```python
from build123d import *

# Parameters (mm, degrees)
SKETCH2_R           = 45.212
SKETCH2_R_2         = 32.258
BOSS_EXTRUDE3_DEPTH = 40.64
SKETCH4_R           = 32.258
BOSS_EXTRUDE4_DEPTH = 7.62
BOSS_EXTRUDE4_TAPER = 25
CUT_EXTRUDE1_DEPTH  = 81.10791158
SKETCH7_R           = 2.286
CUT_EXTRUDE2_DEPTH  = 81.107911519
BOSS_EXTRUDE8_START = -7.62
BOSS_EXTRUDE8_DEPTH = 11.684
SKETCH18_R          = 8.567257543
CUT_EXTRUDE3_DEPTH  = 5.08
SKETCH19_R          = 2.286
CUT_EXTRUDE4_DEPTH  = 85.454467418
BOSS_EXTRUDE9_START = -15.24
BOSS_EXTRUDE9_DEPTH = 15.24
CUT_EXTRUDE5_START  = -28.956
SKETCH21_R          = 2.286
CUT_EXTRUDE5_DEPTH  = 28.956
CIRPATTERN1_COUNT   = 2
CUT_EXTRUDE6_DEPTH  = 91.648631066


with BuildPart() as part:
    # Sketch2 → Boss-Extrude3 (new body)
    # profile 1 of 2: a face of its own
    with BuildSketch(Plane(origin=(0, 0, 0), x_dir=(1, 0, 0), z_dir=(0, 1, 0))):
        with Locations(Location((0, 0, 0), (0, 0, 270))):
            Circle(SKETCH2_R)
        Circle(SKETCH2_R_2, mode=Mode.SUBTRACT)
    # profile 2 of 2: a face of its own
    with BuildSketch(Plane(origin=(0, 0, 0), x_dir=(1, 0, 0), z_dir=(0, 1, 0))):
        Circle(SKETCH2_R_2)
        Polygon((0, 6.35), (-6.35, 3.483506942), (-6.35, -3.483506942), (0, -6.35), (6.35, -3.483506942), (6.35, 3.483506942), align=None, mode=Mode.SUBTRACT)
    extrude(amount=-BOSS_EXTRUDE3_DEPTH)

    # Sketch4 → Boss-Extrude4 (add)
    with BuildSketch(Plane(origin=(0, 0, 0), x_dir=(1, 0, 0), z_dir=(0, 1, 0))):
        Circle(SKETCH4_R)
    extrude(amount=BOSS_EXTRUDE4_DEPTH, taper=BOSS_EXTRUDE4_TAPER)

    # Sketch6 → Cut-Extrude1 (cut, through all)
    with BuildSketch(Plane(origin=(0, -40.64, 0), x_dir=(-1, 0, 0), z_dir=(0, -1, 0))):
        Polygon((6.35, -3.483506942), (0, -6.35), (-6.35, -3.483506942), (-6.35, 3.483506942), (0, 6.35), (6.35, 3.483506942), align=None)
    extrude(amount=-CUT_EXTRUDE1_DEPTH, mode=Mode.SUBTRACT)

    # Sketch7 → Cut-Extrude2 (cut, through all)
    with BuildSketch(Plane(origin=(0, 7.62, 0), x_dir=(1, 0, 0), z_dir=(0, 1, 0))):
        with Locations(Location((-16.495222192, 16.6624, 0), (0, 0, 270))):
            Circle(SKETCH7_R)
        with Locations(Location((16.6624, 16.6624, 0), (0, 0, 270))):
            Circle(SKETCH7_R)
        with Locations(Location((16.6624, -16.6624, 0), (0, 0, 270))):
            Circle(SKETCH7_R)
        with Locations(Location((-16.495222192, -16.6624, 0), (0, 0, 270))):
            Circle(SKETCH7_R)
    extrude(amount=-CUT_EXTRUDE2_DEPTH, mode=Mode.SUBTRACT)

    # Sketch12 → Boss-Extrude8 (add)
    with BuildSketch(Plane(origin=(0, 7.62, 0), x_dir=(1, 0, 0), z_dir=(0, 1, 0)).offset(BOSS_EXTRUDE8_START)):
        with BuildLine():
            ThreePointArc((-45.091998917, -3.291895759), (-45.888251869, -5.330050438), (-47.973633707, -5.992829324))
            ThreePointArc((-47.973633707, -5.992829324), (-61.102572974, -22.2395178), (-40.602051954, -26.246083736))
            ThreePointArc((-40.602051954, -26.246083736), (-38.578530729, -25.413344212), (-36.658465006, -26.462839746))
            ThreePointArc((-36.658465006, -26.462839746), (-42.485382771, -15.46341472), (-45.091998917, -3.291895759))
        make_face()
    extrude(amount=-BOSS_EXTRUDE8_DEPTH)

    # Sketch18 → Cut-Extrude3 (cut)
    with BuildSketch(Plane(origin=(0, 0, 0), x_dir=(1, 0, 0), z_dir=(0, 1, 0))):
        with Locations(Location((-49.645840541, -18.069608212, 0), (0, 0, 270))):
            Circle(SKETCH18_R)
    extrude(amount=-CUT_EXTRUDE3_DEPTH, mode=Mode.SUBTRACT)

    # Sketch19 → Cut-Extrude4 (cut, through all)
    with BuildSketch(Plane(origin=(0, -5.08, 0), x_dir=(1, 0, 0), z_dir=(0, 1, 0))):
        with Locations(Location((-49.645840541, -18.069608212, 0), (0, 0, 270))):
            Circle(SKETCH19_R)
    extrude(amount=-CUT_EXTRUDE4_DEPTH, mode=Mode.SUBTRACT)

    # Sketch20 → Boss-Extrude9 (add)
    with BuildSketch(Plane.XZ.offset(40.64).offset(BOSS_EXTRUDE9_START)):
        with BuildLine():
            ThreePointArc((42.485382852, -15.463414497), (44.831385262, -12.89196184), (48.307822394, -12.717373918))
            Line((48.307822394, -12.717373918), (61.237093085, -17.295868799))
            Line((61.237093085, -17.295868799), (62.000175566, -15.140990351))
            Line((62.000175566, -15.140990351), (60.601893265, -12.209430544))
            Line((60.601893265, -12.209430544), (44.72934622, -6.588666841))
            ThreePointArc((44.72934622, -6.588666841), (43.832551012, -11.082978649), (42.485382852, -15.463414497))
        make_face()
        with BuildLine():
            ThreePointArc((45.180509286, -21.309596065), (42.629626793, -18.941243028), (42.485382852, -15.463414497))
            ThreePointArc((42.485382852, -15.463414497), (40.701683588, -19.684966271), (38.499780526, -23.704257918))
            Line((38.499780526, -23.704257918), (54.271814253, -29.601179693))
            Line((54.271814253, -29.601179693), (57.22733096, -28.254273131))
            Line((57.22733096, -28.254273131), (58.027905034, -26.113040506))
            Line((58.027905034, -26.113040506), (45.180509286, -21.309596065))
        make_face()
    extrude(amount=BOSS_EXTRUDE9_DEPTH)

    # Sketch21 → Cut-Extrude5 (cut)
    # profile 1 of 2: a face of its own
    with BuildSketch(Plane.XZ.offset(40.64).offset(CUT_EXTRUDE5_START)):
        with BuildLine():
            Line((-20.08732464, 27.438707345), (-28.082012675, 35.43339538))
            ThreePointArc((-28.082012675, 35.43339538), (-31.885487137, 32.053715136), (-35.285134805, 28.268077504))
            Line((-35.285134805, 28.268077504), (-27.271504992, 20.254502449))
            Line((-27.271504992, 20.254502449), (-30.86360744, 16.662375455))
            Line((-30.86360744, 16.662375455), (-23.679427089, 9.478195103))
            ThreePointArc((-23.679427089, 9.478195103), (-9.311017295, 9.478195103), (-9.311017295, 23.846604897))
            Line((-9.311017295, 23.846604897), (-16.495222192, 31.030809794))
            Line((-16.495222192, 31.030809794), (-20.08732464, 27.438707345))
        make_face()
        with Locations(Location((-16.495222192, 16.6624, 0), (0, 0, 90))):
            Circle(SKETCH21_R, mode=Mode.SUBTRACT)
    # profile 2 of 2: a face of its own
    with BuildSketch(Plane.XZ.offset(40.64).offset(CUT_EXTRUDE5_START)):
        with BuildLine():
            ThreePointArc((16.6624, 26.8224), (6.5024, 16.6624), (16.6624, 6.5024))
            Line((16.6624, 6.5024), (26.8224, 6.5024))
            Line((26.8224, 6.5024), (26.8224, 11.844066963))
            Line((26.8224, 11.844066963), (43.63304965, 11.844066963))
            ThreePointArc((43.63304965, 11.844066963), (41.873887087, 17.050000709), (39.496151472, 22.004066963))
            Line((39.496151472, 22.004066963), (25.304864582, 22.004066963))
            Line((25.304864582, 22.004066963), (25.304864582, 26.8224))
            Line((25.304864582, 26.8224), (16.6624, 26.8224))
        make_face()
        with Locations(Location((16.6624, 16.6624, 0), (0, 0, 90))):
            Circle(SKETCH21_R, mode=Mode.SUBTRACT)
    cut_extrude5 = extrude(amount=CUT_EXTRUDE5_DEPTH, mode=Mode.SUBTRACT)

    # CirPattern1: Cut-Extrude5 ×2 about axis
    cirpattern1_axis = Axis((0, 0, 0), (0, 1, 0))
    for i in range(1, CIRPATTERN1_COUNT):
        add(cut_extrude5.rotate(cirpattern1_axis, i * 360 / CIRPATTERN1_COUNT), mode=Mode.SUBTRACT)

    # Sketch22 → Cut-Extrude6 (cut, through all)
    with BuildSketch(Plane(origin=(0, 7.62, 0), x_dir=(1, 0, 0), z_dir=(0, 1, 0))):
        Polygon((6.428560964, -3.526604212), (6.268409318, 3.803994999), (-0.160151646, 7.33059921), (-6.428560964, 3.526604212), (-6.268409318, -3.803994999), (0.160151646, -7.33059921), align=None)
    extrude(amount=-CUT_EXTRUDE6_DEPTH, mode=Mode.SUBTRACT)


solid = part.part
```
Can you work these out from the model? Positions are in its coordinate system, mm. A direction names the side the tool comes from. Coordinates: 2 decimals unless noted, no trailing zeros. Loops run counter-clockwise (first coordinate to the right, second up) from the corner with the lowest first, then second, coordinate; pieces in that order, holes last.
Item 1: If we mould it in two halves opening along Z, with no side actions, what happens to faces 5 (the face through (12.853, -25.959, -27.388)), 6 (the face through (61.311, -32.913, -13.696))? For each: released by +Z, released by -Z, zero draft, split by the parting line, or undercut.
Answers below:
face 5: undercut
face 6: released by +Z
Item 2: I'm going to push flat-ended pins straight in: pin 1 (11 mm diameter, centred on x = -22, y = -19.5, fed in from -Z); pin 2 (1 mm diameter, centred on x = -25.5, z = 26.5, fed in from +Y); pin 3 (2 mm diameter, centred on y = -11.5, z = 1, fed in from -X); pin 4 (4 mm diameter, centred on x = -49.65, z = 18.07, fed in from +Y). Where does each tip first touch, or does it pass through?
Answers below:
pin 1: stops at z = -42.09
pin 2: stops at y = 0
pin 3: stops at x = -45.21
pin 4: passes through
Item 3: Which directions (+Z, -Z, +X, -X, +Y, -Y) give clear straight access to the entire face, cutting with the end or side of a thin tool? Please do faces 1 (the face through (35, -26, 11.844)), 2 (the face through (-6.35, -17, 2)), 3 (the face through (-51.4, -5.08, 19.9)), 4 (the face through (-26.822, -26, -9)).
Answers below:
face 1: +X, -Y
face 2: +Y, -Y
face 3: +Y
face 4: -Y
Item 4: Please list where these lines run through material, in increasing order: L1, parallel to Z at x = 19, y = -12.5; L2, parallel to Z at x = 30, y = -35.5; L3, parallel to X at y = 2, z = 18.5 (3 decimals).
Answers below:
L1: z = -41.03 to -28.53, -6.82 to 6.5, 26.82 to 41.03
L2: z = -22.98 to -17.53, -15.8 to 11.84, 22 to 33.82
L3: x = -25.279 to -17.855, -15.135 to 15.303, 18.022 to 25.279
Item 5: Suppose I cut it at B-B (z = -37). Please give me the cut outline in (x, y).
Answers below:
outline: (-25.98, -40.64) - (25.98, -40.64) - (25.98, 0) - (-25.98, 0) - close
Item 6: Suppose I cut it at A-A (y = -23.5). State how many separate pieces and enclosed holes the cut face has, then the cut area to 3 significant figures.
Answers below:
separate pieces: 3
enclosed holes: 1
area: 4,290 mm2
